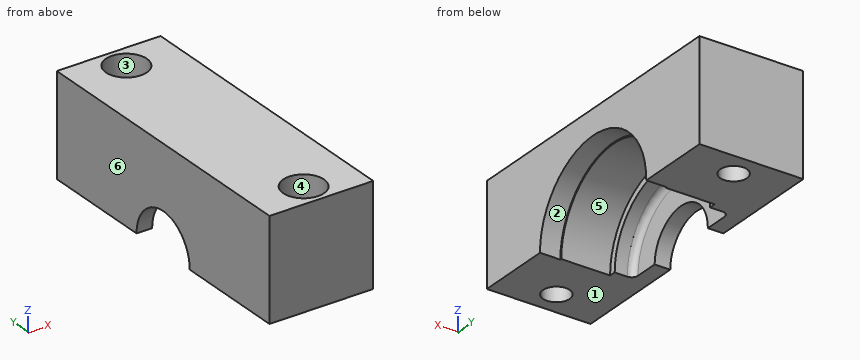
from build123d import *

# Parameters (mm, degrees)
F1_DEPTH        = 52.324
F2_R            = 38.1
F3_DEPTH        = 104.649
F4_R            = 68.326
F5_DEPTH        = 88.9
F6_R            = 6.35
F7_R            = 74.93
F8_DEPTH        = 69.85
F9_R            = 76.2
F10_DEPTH       = 20.574
F12_D           = 26.924
F12_CBORE_D     = 41.275
F12_CBORE_DEPTH = 26.924


with BuildPart() as f1:
    # F0 (on Right) → F1 (new body, symmetric)
    with BuildSketch(Plane.YZ):
        Polygon((-152.4, 0), (0, 0), (152.4, 0), (152.4, 101.6), (0, 101.6), (-152.4, 101.6), align=None)
    extrude(amount=F1_DEPTH, both=True)

    # F2 (on face) → F3 (cut, through all)
    with BuildSketch(Plane.YZ.offset(52.324)):
        Circle(F2_R)
    extrude(amount=-F3_DEPTH, mode=Mode.SUBTRACT)

    # F4 (on face) → F5 (cut)
    with BuildSketch(Plane.YZ.offset(52.324)):
        Circle(F4_R)
    extrude(amount=-F5_DEPTH, mode=Mode.SUBTRACT)

    # F6
    f6_edges = [f1.edges().sort_by_distance(p)[0] for p in [
        (-36.576, 0, 68.326),
    ]]
    fillet(f6_edges, radius=F6_R)

    # F7 (on face) → F8 (cut)
    with BuildSketch(Plane.YZ.offset(52.324)):
        Circle(F7_R)
    extrude(amount=-F8_DEPTH, mode=Mode.SUBTRACT)

    # F9 (on face) → F10 (cut)
    with BuildSketch(Plane.YZ.offset(52.324)):
        Circle(F9_R)
    extrude(amount=-F10_DEPTH, mode=Mode.SUBTRACT)

    # F12 (through all)
    with Locations(Plane.XY.offset(101.6)):
        with Locations((0, -127), (0, 127)):
            CounterBoreHole(F12_D / 2, F12_CBORE_D / 2, F12_CBORE_DEPTH)


solid = f1.part
CAD build for the part. Positions are in the model's coordinates, mm. Face numbers are marked on the shaded views. A direction names the side the tool comes from. Coordinates: 2 decimals unless noted, no trailing zeros. Write each loop counter-clockwise with the first axis right and the second up, starting at its lowest first coordinate (ties: lowest second). Pieces come first, ordered by that corner, then holes. Notation, with made-up numbers: (-9, 5) - (27, 5) arc R11 cw to (27, 23) - close; hole circle Ø9 at (-21.75, -37). An arc over 180 degrees is marked (long way). Use a Markdown table: item, result. Add a question column.
Item 1: Band-saw the part on D-D, the plane z = 90.5. Give the cut face in (x, y) (1 decimal), and give its area (3 significant figures).
Item 2: Drill centre lines: L1, parallel to Y at x = 0, z = 87; L2, parallel to Y at x = -15, z = 88; L3, parallel to Y at x = 0, z = 58. Where is each one in solid material? Low to high. Write a range as from..to.
Item 3: Band-saw the part on C-C, the plane y = 0. Give the cut face in (x, z), and give its area (3 significant figures).
Item 4: Band-saw the part on B-B, the plane x = 0. Give the cut face in (y, z).
Item 5: Band-saw the part on A-A, the plane y = -127. Give the cut face in (x, z), and give its area (3 significant figures).
Item 6: 3-axis set-ups, long thin cutter, end or side, ignore diameter. For the marked faces 1, 2 and 3: which of +Z, -Z, +X, -X, +Y, -Y reach the whole face in a straight line?
Item 7: Mould opens along X. For the marked faces 4, 5 and 6 say: pulls with the +X half, pulls with the -X half, needs draft (parallel to the pull), parting line crosses it, or undercut.
Item 8: Flat gauge pins, fed straight in: pin 1 (1 mm diameter, centred on x = 14, y = 16.5, fed in from -Z); pin 2 (12.5 mm diameter, centred on x = 10, y = -118.5, fed in from +Z); pin 3 (8 mm diameter, centred on x = -30, y = 50, fed in from -Z). Where does each tip first touch, or does it go through?
Numbers:
| question | item | result |
|---|---|---|
| 1 | outline | (-52.3, -152.4) - (52.3, -152.4) - (52.3, 152.4) - (-52.3, 152.4) - close; hole circle Ø41.3 at (0, -127); hole circle Ø41.3 at (0, 127) |
| 1 | area | 29,200 mm2 |
| 2 | L1 | -152.4..-147.64, -106.36..106.36, 147.64..152.4 |
| 2 | L2 | -152.4..-141.17, -112.83..112.83, 141.17..152.4 |
| 2 | L3 | -152.4..-140.46, -113.54..-47.44, 47.44..113.54, 140.46..152.4 |
| 3 | outline | (-52.32, 38.1) - (-36.58, 38.1) - (-36.58, 61.98) arc R6.35 cw to (-30.23, 68.33) - (-17.53, 68.33) - (-17.53, 74.93) - (31.75, 74.93) - (31.75, 76.2) - (52.32, 76.2) - (52.32, 101.6) - (-52.32, 101.6) - close |
| 3 | area | 3,480 mm2 |
| 4 | outline | (-152.4, 0) - (-140.46, 0) - (-140.46, 74.68) - (-147.64, 74.68) - (-147.64, 101.6) - (-152.4, 101.6) - close; (-113.54, 0) - (-74.93, 0) arc R74.93 cw to (74.93, 0) - (113.54, 0) - (113.54, 74.68) - (106.36, 74.68) - (106.36, 101.6) - (-106.36, 101.6) - (-106.36, 74.68) - (-113.54, 74.68) - close; (140.46, 0) - (152.4, 0) - (152.4, 101.6) - (147.64, 101.6) - (147.64, 74.68) - (140.46, 74.68) - close |
| 5 | outline | (-52.32, 0) - (-13.46, 0) - (-13.46, 74.68) - (-20.64, 74.68) - (-20.64, 101.6) - (-52.32, 101.6) - close; (13.46, 0) - (52.32, 0) - (52.32, 101.6) - (20.64, 101.6) - (20.64, 74.68) - (13.46, 74.68) - close |
| 5 | area | 7,510 mm2 |
| 6 | face 1 | -Z, +X, -X, +Y, -Y |
| 6 | face 2 | -Z, +X |
| 6 | face 3 | +Z |
| 7 | face 4 | undercut |
| 7 | face 5 | needs draft |
| 7 | face 6 | pulls with the -X half |
| 8 | pin 1 | z = 72.98 |
| 8 | pin 2 | z = 74.68 |
| 8 | pin 3 | z = 41.86 |
